Geometry: final body of the model. Coordinates: model frame, mm. A direction names the side the tool comes from. Give positions to 0.01 mm unless a question says otherwise; leave off trailing zeros. Order: outer loops, then holes, each group sorted by start corner. A loop starts at its lowest first (then second) coordinate and runs counter-clockwise, first axis right, second up. Notation, with made-up numbers: M 32,-38 L 90,-38 A6 ccw 90,-32 Z; hole C 62.5,-27.5 d5. An arc over 180 degrees is marked long. One line per item, written item: value. Start each with the question number.
```python
from build123d import *

# Parameters (mm, degrees)
EXTRUDE_4_DEPTH     = 15
SKETCH_3_R          = 10.1
CUT_EXTRUDE_1_DEPTH = 2


with BuildPart() as part:
    # ｽｹｯﾁ2 → ﾎﾞｽ - 押し出し4 (new body)
    with BuildSketch(Plane(origin=(0, 0, 0), x_dir=(1, 0, 0), z_dir=(0, 1, 0))):
        with BuildLine():
            ThreePointArc((-53.82643789, -36.437818048), (-56.846261527, -34.367935813), (-60.466933112, -34.910600109))
            Line((-60.466933112, -34.910600109), (-64.807406984, -37.416573868))
            ThreePointArc((-64.807406984, -37.416573868), (-67.177509772, -40.614402853), (-66.461234116, -44.529814279))
            ThreePointArc((-66.461234116, -44.529814279), (49.665387485, -62.716419588), (58.57572973, 54.487465409))
            Line((58.57572973, 54.487465409), (57.289371136, 55.838409315))
            Line((57.289371136, 55.838409315), (25.911523347, 88.791671712))
            ThreePointArc((25.911523347, 88.791671712), (19.306695871, 93.382511176), (11.427401304, 95))
            Line((11.427401304, 95), (0, 95))
            ThreePointArc((0, 95), (-15, 80), (0, 65))
            ThreePointArc((0, 65), (57.41714976, -30.467538684), (-53.82643789, -36.437818048))
        make_face()
    extrude(amount=EXTRUDE_4_DEPTH)

    # ｽｹｯﾁ3 → ｶｯﾄ - 押し出し1 (cut)
    with BuildSketch(Plane.XZ):
        with Locations(Location((0, -80, 0), (0, 0, 270))):
            Circle(SKETCH_3_R)
    extrude(amount=-CUT_EXTRUDE_1_DEPTH, mode=Mode.SUBTRACT)


solid = part.part
```
Q1. Section query A-A on y = 12.5. Return loops of the section in (x, z).
Q2. Section query B-B on z = 41. Return loops of the section in (x, y).
Q3. Set-up query: faces 1 (the face through (0, 2, -80)), 2 (the face through (66, 15, 5)). Return all of +Z, -Z, +X, -X, +Y, -Y with unobstructed straight access to the full face (end or side cutting, diameter ignored); none if empty.
Q4. Contact query for flat-ended pins moving along their axis: pin 1 (8 mm diameter, centred on x = 47, y = 4, fed in from +Z); pin 2 (6 mm diameter, centred on y = 7.5, z = -16.5, fed in from +X); pin 3 (6 mm diameter, centred on y = 11, z = -32, fed in from +X). Output: stop coordinate, or through.
Q5. Section query C-C on x = 14. Return loops of the section in (y, z), and give its area (3 significant figures).
Q6. Ray query, line 1 along X through (y, z) = (0.4, -80); line 2 along Z through (x, y) = (0, 10); line 3 along Z through (x, y) = (38.5, 13.5). Return the intervals inside material, ascending. Write a range as [from, to].
Q7. Mould query, pull axis X, two halves, no side actions, for faces 3 (the face through (-67.164, 7.395, 40.559)), 4 (the face through (-56.8, 7.4, 34.38)), 5 (the face through (6, 7, -95)). Classes: +X half, -X half, draft (parallel to the pull), parting line (faces both ways), or undercut.
Q8. Section query D-D on z = -80. Return loops of the section in (x, y), and give its area (3 significant figures).
Results below:
1. outline: M -66.46,44.53 A5 ccw -64.81,37.42 L -60.47,34.91 A5 ccw -53.83,36.44 A65 cw long 0,-65 A15 ccw 0,-95 L 11.43,-95 A20 ccw 25.91,-88.79 L 58.58,-54.49 A80 ccw long Z
2. outline: M -67.25,0 L -50.44,0 L -50.44,15 L -67.25,15 Z; M 50.44,0 L 68.69,0 L 68.69,15 L 50.44,15 Z
3. face 1: -Y
3. face 2: +Z, -Z, +X, -X, +Y
4. pin 1: z = 67.46
4. pin 2: x = 78.85
4. pin 3: x = 74.56
5. outline: M 0,-94.83 L 15,-94.83 L 15,-63.47 L 0,-63.47 Z; M 0,63.47 L 15,63.47 L 15,78.77 L 0,78.77 Z
5. area: 700 mm2
6. line 1: [-15, -10.1], [10.1, 34.28]
6. line 2: [-95, -65], [65, 80]
6. line 3: [-75.57, -52.37], [52.37, 70.13]
7. face 3: -X half
7. face 4: undercut
7. face 5: draft
8. outline: M -15,0 L -10.1,0 L -10.1,2 L 10.1,2 L 10.1,0 L 34.28,0 L 34.28,15 L -15,15 Z
8. area: 699 mm2
